Design review of the part built by this model. Coordinates are the model's own, in mm. Coordinates: 2 decimals unless noted, no trailing zeros. Loops run counter-clockwise (first coordinate to the right, second up) from the corner with the lowest first, then second, coordinate; pieces in that order, holes last. Notation, with made-up numbers: (61, 48) - (99, 48) arc R15 cw to (99, 77) - close; hole circle Ø11 at (64.5, 69.5). An arc over 180 degrees is marked (long way). Answer in a Markdown table with one row per item. Add a question column.
(1) To check wall thickness, follow L1, parallel to Y at x = -39.5, z = 1583.5; L2, parallel to X at y = -57, z = 1613.5; L3, parallel to Y at x = -23, z = 1918. State the ranges of each line that lie inside material, in increasing order. Write a range as [from, to].
(2) We need section A-A, the plane x = 94.5. Write out the cut boundary in (y, z), plus the area to 3 significant figures.
(3) We need section C-C, the plane y = -97. Write out the cut boundary in (x, z), plus the area to 3 significant figures.
(4) We need section B-B, the plane z = 2018.5. Write out the cut boundary in (x, y), plus the area to 3 significant figures.
(5) Clearance check with flat-ended pins moving along their axes: pin 1 (3 mm diameter, centred on y = -133.5, z = 544, fed in from +X); pin 2 (8 mm diameter, centred on y = 112.5, z = 994.5, fed in from +X); pin 3 (4 mm diameter, centred on y = -134, z = 1571.5, fed in from +X). State where each tip first meets the part, or that it passes through.
Autodesk Inventor part; units mm, degrees
ref_plane "Start plane" through (0, 0, 0) normal (0, 0, 1) x (1, 0, 0)
ref_plane "End plane" through (0, 0, 2620) normal (0, 0, 1) x (1, 0, 0)
ref_plane "YZ Plane" through (0, 0, 0) normal (1, 0, 0) x (0, 1, 0)
ref_plane "Start plane" through (0, 0, 0) normal (0, 0, 1) x (1, 0, 0)
ref_plane "End plane" through (0, 0, 2620) normal (0, 0, 1) x (1, 0, 0)
sketch "Sketch" plane through (0, 0, 0) normal (0, 0, 1) x (1, 0, 0)
  line L0 (-161, -182.5) -> (-161, -138.4)
  line L1 (-161, -138.4) -> (-28.65, -138.4)
  line L2 (-13.45, -123.2) -> (-13.45, 0)
  line L3 (-13.45, 0) -> (0, 0) construction
  line L4 (0, 0) -> (0, -182.5) construction
  line L5 (0, -182.5) -> (-161, -182.5)
  line L6 (-60, 0) -> (80, 0) construction
  line L7 (0, -60) -> (0, 80) construction
  line L8 (161, -182.5) -> (161, -138.4)
  line L9 (161, -138.4) -> (28.65, -138.4)
  line L10 (13.45, -123.2) -> (13.45, 0)
  line L11 (13.45, 0) -> (0, 0) construction
  line L12 (0, -182.5) -> (161, -182.5)
  line L13 (-161, 182.5) -> (-161, 138.4)
  line L14 (-161, 138.4) -> (-28.65, 138.4)
  line L15 (-13.45, 123.2) -> (-13.45, 0)
  line L16 (0, 182.5) -> (-161, 182.5)
  line L17 (161, 182.5) -> (161, 138.4)
  line L18 (161, 138.4) -> (28.65, 138.4)
  line L19 (0, 182.5) -> (161, 182.5)
  line L20 (13.45, 123.2) -> (13.45, 0)
  arc A0 (-13.45, 123.2) -> (-28.65, 138.4) centre (-28.65, 123.2) ccw
  arc A1 (28.65, 138.4) -> (13.45, 123.2) centre (28.65, 123.2) ccw
  arc A2 (13.45, -123.2) -> (28.65, -138.4) centre (28.65, -123.2) ccw
  arc A3 (-28.65, -138.4) -> (-13.45, -123.2) centre (-28.65, -123.2) ccw
  line L21 (0, 108) -> (0, -88) construction
  line L22 (-88, 0) -> (108, 0) construction
  point P0 (-13.45, -138.4)
  point P1 (13.45, -138.4)
  point P2 (-13.45, 138.4)
  point P3 (13.45, 138.4)
  dimension "d1" = 182.5
  dimension "d2" = 44.1
  dimension "d3" = 161
  dimension "d4" = 13.45
  dimension "d10" = 15.2
extrude "Body" add sketch "Sketch" along normal up to surface (2620 mm away) from surface at 0
sketch "Sketch4" plane through (0, 0, 0) normal (0, 0, 1) x (1, 0, 0)
  line L0 (0, 0) -> (10, 0)
ref_plane "Work Plane3" through (0, 0, 0) normal (0, -1, 0) x (1, 0, 0)
sketch "Sketch5" plane through (0, 0, 0) normal (0, -1, 0) x (1, 0, 0)
  line L0 (-2, 0) -> (12, 0)
  line L1 (-2, 2620) -> (12, 2620)
  dimension "d14" = 2620
equation "\"d1\" = 0.5 * G_H"
equation "\"d2\" = G_T1"
equation "\"d3\" = 0.5 * G_W"
equation "\"d4\" = 0.5 * G_T"
equation "\"d10\" = G_IR"
equation "\"d5\" = G_L"
equation "\"G_W\" = 322"
equation "\"G_H\" = 365"
equation "\"G_T\" = 26.9"
equation "\"G_T1\" = 44.1"
equation "\"G_IR\" = 15.2"
equation "\"G_L\" = d14"
equation "\"G_OFFSET_START\" = 0"
equation "\"G_OFFSET_END\" = 0"
properties part number "AS 3679 - 310 UC - 283 - 2620" material "Steel, Mild"
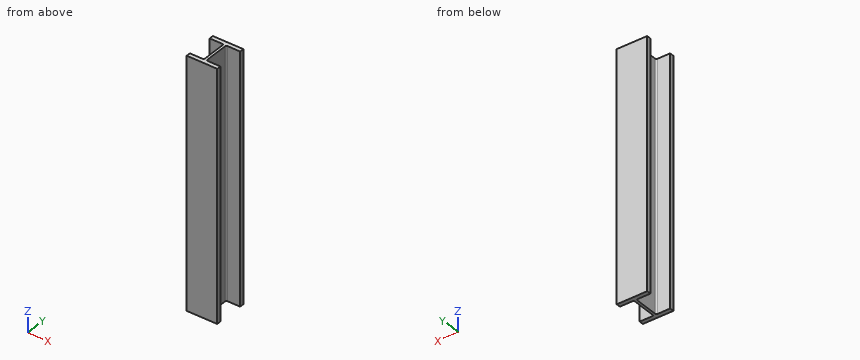
Responses:
| question | item | result |
|---|---|---|
| 1 | L1 | y = [-182.5, -138.4], [138.4, 182.5] |
| 1 | L2 | x = [-13.45, 13.45] |
| 1 | L3 | y = [-182.5, -137.31], [137.31, 182.5] |
| 2 | outline | (-182.5, 0) - (-138.4, 0) - (-138.4, 2620) - (-182.5, 2620) - close; (138.4, 0) - (182.5, 0) - (182.5, 2620) - (138.4, 2620) - close |
| 2 | area | 231,000 mm2 |
| 3 | outline | (-13.45, 0) - (13.45, 0) - (13.45, 2620) - (-13.45, 2620) - close |
| 3 | area | 70,500 mm2 |
| 4 | outline | (-161, -182.5) - (161, -182.5) - (161, -138.4) - (28.65, -138.4) arc R15.2 cw to (13.45, -123.2) - (13.45, 123.2) arc R15.2 cw to (28.65, 138.4) - (161, 138.4) - (161, 182.5) - (-161, 182.5) - (-161, 138.4) - (-28.65, 138.4) arc R15.2 cw to (-13.45, 123.2) - (-13.45, -123.2) arc R15.2 cw to (-28.65, -138.4) - (-161, -138.4) - close |
| 4 | area | 36,000 mm2 |
| 5 | pin 1 | stops at x = 19.07 |
| 5 | pin 2 | stops at x = 13.45 |
| 5 | pin 3 | stops at x = 20.45 |
